Model file for the job. Use its own axes, mm. Face numbers are marked on the shaded views. A direction names the side the tool comes from. Give positions to 0.01 mm unless a question says otherwise; leave off trailing zeros. Write each loop counter-clockwise with the first axis right and the second up, starting at its lowest first coordinate (ties: lowest second). Pieces come first, ordered by that corner, then holes. Notation, with made-up numbers: M 9.5,-14.75 L 51.5,-14.75 A32 ccw 51.5,23.25 Z; hole C 17.25,18 d10. An arc over 180 degrees is marked long. Answer as a JSON object with one key per item and string values. Group by question number.
```python
from build123d import *

# Parameters (mm, degrees)
F1_DEPTH = 20
F2_R     = 2
F3_R     = 2
F4_DEPTH = 25
F5_R     = 9.99999


# Not quite as in the source:
# - a fillet or chamfer is up to 0.001 mm smaller than in the source, because OpenCascade refuses the exact size


with BuildPart() as f1:
    # F0 (on Front) → F1 (new body)
    with BuildSketch(Plane.XZ):
        with BuildLine():
            Line((0, 3), (0, 0))
            Line((0, 0), (60, 0))
            Line((60, 0), (60, 3))
            Line((60, 3), (39.9215674165, 3))
            ThreePointArc((39.9215674165, 3), (44.9926379155, 13.7800975251), (40.6066017178, 24.8566017178))
            Line((40.6066017178, 24.8566017178), (37.9549512883, 22.2049512883))
            ThreePointArc((37.9549512883, 22.2049512883), (30, 3), (22.0450487117, 22.2049512883))
            Line((22.0450487117, 22.2049512883), (19.3933982822, 24.8566017178))
            ThreePointArc((19.3933982822, 24.8566017178), (15.0073620845, 13.7800975251), (20.0784325835, 3))
            Line((20.0784325835, 3), (0, 3))
        make_face()
    extrude(amount=F1_DEPTH)

    # F2
    f2_edges = [f1.edges().sort_by_distance(p)[0] for p in [
        (22.045049, -10, 22.204951),
        (37.954951, -10, 22.204951),
    ]]
    fillet(f2_edges, radius=F2_R)

    # F3 (on face) → F4 (cut)
    with BuildSketch(Plane.XY.offset(3)):
        with Locations((6, -10)):
            Circle(F3_R)
        with Locations((54, -10)):
            Circle(F3_R)
    extrude(amount=-F4_DEPTH, mode=Mode.SUBTRACT)

    # F5 (radius 10 in the source; OpenCascade refuses exactly that, so slightly less here)
    f5_edges = [f1.edges().sort_by_distance(p)[0] for p in [
        (0, 0, 1.5),
        (0, -20, 1.5),
        (60, -20, 1.5),
        (60, 0, 1.5),
    ]]
    fillet(f5_edges, radius=F5_R)


solid = f1.part
```
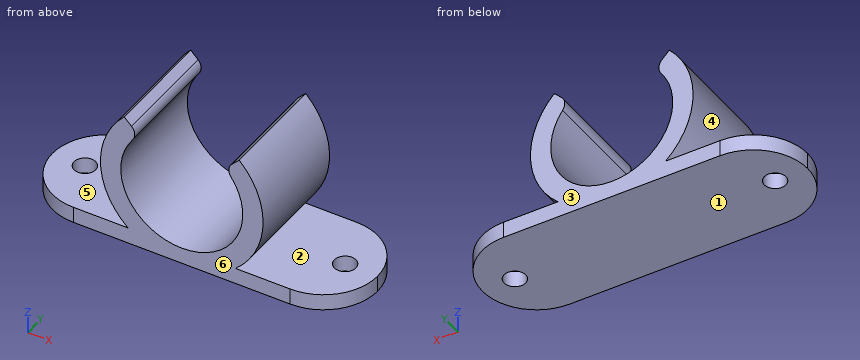
Q1. Drop flat-ended pins along their axis: P1, Ø4, axis at x = 47.5, y = -5, coming from the +Z side; P2, Ø5, axis at x = 24.5, y = -12.5, coming from the +Z side; P3, Ø12, axis at y = -17.5, z = 3.5, coming from the -X side. Give the stop position or say it passes through.
Q2. Two-plate mould, pull along Z, no slides. Class the marked faces 1, 2, 3 and 4: +Z half, -Z half, draft (parallel to the pull), parting line (faces both ways), or undercut.
Q3. Slice it at C-C, the plane z = 1.75. Count the separate pieces of the cut face and the enclosed holes in it, then the cut area to 3 significant figures.
Q4. Slice it at A-A, the plane z = 17. Write the cut outline in (x, y), then the cut area to 3 significant figures.
Q5. Slice it at B-B, the plane x = 54. Write the cut outline in (y, z), then the cut area to 3 significant figures.
Q6. Wall check: L1, parallel to X at y = -14.25, z = 14.25; L2, parallel to X at y = -8.75, z = 1.5; L3, parallel to Z at x = 9.5, y = -7.5. Give the ranges that are in metal, low to high.
Q7. Slice it at D-D, the plane y = -11. Write the cut outline in (x, z).
Q8. 3-axis set-ups, long thin cutter, end or side, ignore diameter. For the marked faces 5 and 6: which of +Z, -Z, +X, -X, +Y, -Y reach the whole face in a straight line?
Solved:
{
 "1": {"P1": "stops at z = 3", "P2": "stops at z = 6.34", "P3": "stops at x = 0.12"},
 "2": {"face 1": "-Z half", "face 2": "undercut", "face 3": "draft", "face 4": "undercut"},
 "3": {"separate pieces": "1", "enclosed holes": "2", "area": "1,090 mm²"},
 "4": {"outline": "M 15.25,-20 L 19.09,-20 L 19.09,0 L 15.25,0 Z; M 40.91,-20 L 44.75,-20 L 44.75,0 L 40.91,0 Z", "area": "153 mm²"},
 "5": {"outline": "M -19.17,0 L -12,0 L -12,3 L -19.17,3 Z; M -8,0 L -0.83,0 L -0.83,3 L -8,3 Z", "area": "43.0 mm²"},
 "6": {"L1": "x = 15 to 18.75, 41.25 to 45", "L2": "x = 0.08 to 4.44, 7.56 to 52.44, 55.56 to 59.92", "L3": "z = 0 to 3"},
 "7": {"outline": "M 0.05,0 L 4.27,0 L 4.27,3 L 0.05,3 Z; M 7.73,0 L 52.27,0 L 52.27,3 L 39.92,3 A15 ccw 40.61,24.86 L 39.26,23.51 A2 ccw 39.06,20.91 A11.25 cw long 20.94,20.91 A2 ccw 20.74,23.51 L 19.39,24.86 A15 ccw 20.08,3 L 7.73,3 Z; M 55.73,0 L 59.95,0 L 59.95,3 L 55.73,3 Z"},
 "8": {"face 5": "-X, +Y, -Y", "face 6": "+Z, -Z, +X, -X, -Y"}
}
